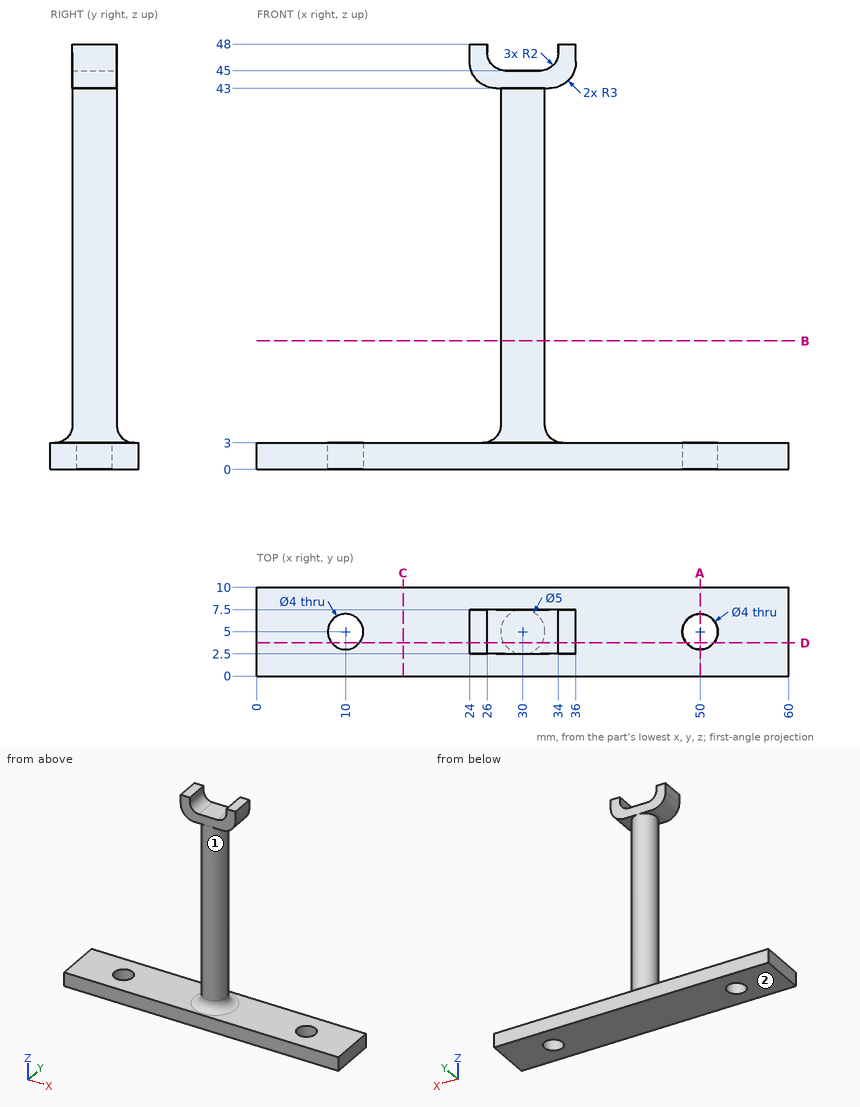
Design review of the part shown in the three views and the two pictorial views. Dimensions are in mm from the part's minimum x, y and z. Round coordinates to 2 decimals unless told otherwise and drop trailing zeros. Loops run counter-clockwise (first coordinate to the right, second up) from the corner with the lowest first, then second, coordinate; pieces in that order, holes last. Notation, with made-up numbers: M -0.5,-13.75 L 3.5,-13.75 A11 cw 3.5,0.25 Z; hole C -5,17.25 d6. An arc over 180 degrees is marked long. Write item = value, one per line.
Item 1: For line 1 (Y direction, x = 10, z = 1.1); line 2 (Y direction, x = 31.5, z = 18); line 3 (X direction, y = 6.5, z = 9.5), list the stretches that pass through material, from the lowest coordinate up. Write a range as [from, to].
Return value:
line_1 = [0, 3], [7, 10]
line_2 = [3, 7]
line_3 = [28, 32]
Item 2: Insertion check: P1, Ø2.5, axis at x = 32, z = 46.5, coming from the +Y side; P2, Ø0.8, axis at y = 4, z = 47.5, coming from the +X side; P3, Ø5, axis at y = 3, z = 27.5, coming from the -X side; P4, Ø4, axis at x = 31.5, z = 41, coming from the -Y side. Each pin has a flat end and moves straight along its axis. Give the tip position at first contact, or say it passes through.
Return value:
P1 = through
P2 = 36
P3 = 27.5
P4 = 2.5
Item 3: Take a section at B-B on z = 14.5. Write out the cut boundary in (x, y), then the cut area to 3 significant figures.
Return value:
outline = C 30,5 d5
area = 19.6 mm2
Item 4: Take a section at D-D on y = 3.75. State how many separate pieces and enclosed holes the cut face has, then the cut area to 3 significant figures.
Return value:
separate_pieces = 3
enclosed_holes = 0
area = 370 mm2
Item 5: Take a section at C-C on x = 16.5. Write out the cut boundary in (y, z).
Return value:
outline = M 0,0 L 10,0 L 10,3 L 0,3 Z
Item 6: Take a section at A-A on x = 50. Write out the cut boundary in (y, z).
Return value:
outline = M 0,0 L 3,0 L 3,3 L 0,3 Z; M 7,0 L 10,0 L 10,3 L 7,3 Z
Item 7: The part is to be moulded in two halves that separate along Z. For the marked faces 1 and 2, say which applies: released by +Z, released by -Z, zero draft, split by the parting line, or undercut.
Return value:
face_1 = undercut
face_2 = released by -Z
